CAD build for the part. Positions are in the model's coordinates, mm. Face numbers are marked on the shaded views. A direction names the side the tool comes from. Coordinates: 2 decimals unless noted, no trailing zeros. Loops run counter-clockwise (first coordinate to the right, second up) from the corner with the lowest first, then second, coordinate; pieces in that order, holes last.
1) Which spindle directions (+Z, -Z, +X, -X, +Y, -Y) get a long thin tool onto all of the face, cutting with end or side? Do the marked faces 1 and 2. Say none if no direction does.
2) Saw through at A-A, the plane z = 0. Write the cut outline in (x, y), and give its area (3 significant figures).
3) Wall check: line 1 along X through (y, z) = (7, 0.25); line 2 along X through (y, z) = (3.25, -5); line 3 along Z through (x, y) = (-4.25, 7.5). Give the ranges that are in metal, low to high.
4) Pin check, flat tips, straight feed: pin 1 Ø2 at (x, y) = (5.5, 3) entering from +Z; pin 2 Ø1 at (y, z) = (4.5, -5) entering from +X; pin 3 Ø6 at (y, z) = (2, -0.5) entering from +X. Stop position of each tip, or through.
5) Saw through at B-B, the plane x = 0. Write the cut outline in (y, z), and give its area (3 significant figures).
6) Saw through at C-C, the plane y = 5. Write the cut outline in (x, z), and give its area (3 significant figures).
7) Saw through at D-D, the plane z = 6.5. Write the cut outline in (x, y).
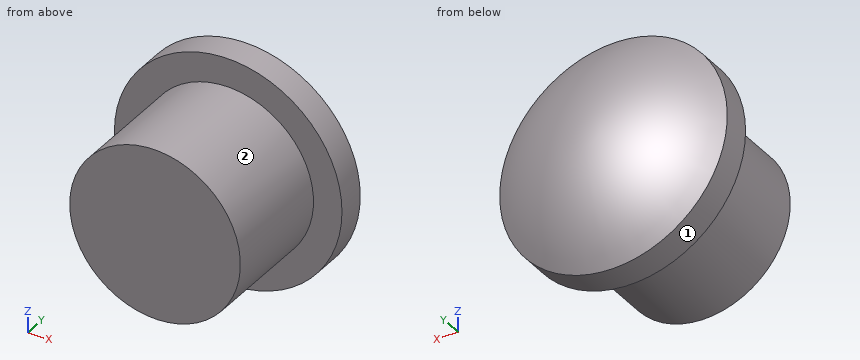
Autodesk Inventor part; units mm, degrees
ref_plane "YZ Plane" through (0, 0, 0) normal (1, 0, 0) x (0, 1, 0)
ref_plane "XZ Plane" through (0, 0, 0) normal (0, 1, 0) x (-1, 0, 0)
ref_plane "XY Plane" through (0, 0, 0) normal (0, 0, 1) x (1, 0, 0)
sketch "Sketch1" plane through (0, 0, 0) normal (0, 1, 0) x (-1, 0, 0)
  circle A0 centre (0, 0) radius 6
  dimension "d0" = 12
extrude "Extrusion1" add sketch "Sketch1" along normal blind 8
sketch "Sketch2" plane through (0, 8, 0) normal (0, 1, 0) x (1, 0, 0)
  circle A0 centre (0, 0) radius 8
  dimension "d3" = 16
extrude "Extrusion2" add sketch "Sketch2" along normal blind 5
sketch "Sketch3" plane through (0, 0, 0) normal (1, 0, 0) x (0, 1, 0)
  line L0 (13, -8) -> (13, 8)
  line L1 (8, -8) -> (8, 8)
  line L2 (8, 8) -> (13, 8)
  line L3 (8, -8) -> (13, -8)
  line L4 (8, 8) -> (10, 8)
  line L5 (10, 8) -> (10, 0)
  line L6 (10, 0) -> (13, 0)
  line L7 (13, -8) -> (13, 8)
  line L8 (10, 0) -> (10, -8)
  arc A0 (10, -8) -> (10, 8) centre (0.8333, 0) ccw
  point P0 (0, 0)
  dimension "d6" = 2
revolve "Revolution1" cut sketch "Sketch3" angle 360 about axis through (0, 10, 0) along (0, 1, 0) contours L3 A0 L0 | A0 L2 L0
properties part number "lense"
Data:
1. face 1: +Y, -Y
1. face 2: -Y
2. outline: (-8, 8) - (-6, 8) - (-6, 0) - (6, 0) - (6, 8) - (8, 8) - (8, 10) arc R12.17 ccw to (-8, 10) - close
2. area: 161 mm2
3. line 1: x = -5.99 to 5.99
3. line 2: x = -3.32 to 3.32
3. line 3: z = -4.24 to 4.24
4. pin 1: stops at z = 3.97
4. pin 2: stops at x = 3.97
4. pin 3: stops at x = 6
5. outline: (0, -6) - (8, -6) - (8, -8) - (10, -8) arc R12.17 ccw to (10, 8) - (8, 8) - (8, 6) - (0, 6) - close
5. area: 161 mm2
6. outline: circle Ø12 at (0, 0)
6. area: 113 mm2
7. outline: (-4.66, 8) - (4.66, 8) - (4.66, 10) arc R10.28 ccw to (-4.66, 10) - close
